Build history of the part. All positions in model axes, mm. Face numbers are marked on the shaded views. A direction names the side the tool comes from. Round coordinates to 2 decimals unless told otherwise and drop trailing zeros. Write each loop counter-clockwise with the first axis right and the second up, starting at its lowest first coordinate (ties: lowest second). Pieces come first, ordered by that corner, then holes. Notation, with made-up numbers: (68, 34) - (108, 34) arc R33 cw to (108, 70) - close; hole circle Ø2 at (14.25, 50.25). An arc over 180 degrees is marked (long way). Answer as a JSON object with one key per item and string values. Group by question number.
Item 1: Probe line 1 (Y direction, x = 9.5, z = 16); line 2 (Z direction, x = 2.25, y = -17.5); line 3 (Z direction, x = 8, y = -4). List the from-to ranges inside material, lowest first. Write a range as from..to.
Item 2: Two-plate mould, pull along Y, no slides. Class the marked faces 3, 4, 5 and 6: +Y half, -Y half, draft (parallel to the pull), parting line (faces both ways), or undercut.
Item 3: Slice it at A-A, the plane z = 16. List the corners of the cut face in (x, y).
Item 4: Which spindle directions (+Z, -Z, +X, -X, +Y, -Y) get a long thin tool onto all of the face, cutting with end or side? Do the marked faces 1 and 2. Say none if no direction does.
Item 5: Flat gauge pins, fed straight in: pin 1 (3.5 mm diameter, centred on x = 7.5, y = -6.5, fed in from +Z); pin 2 (1.5 mm diameter, centred on y = -16, z = -11, fed in from -X). Where does each tip first touch, or does it go through?
Item 6: Slice it at B-B, the plane y = -17. List the corners of the cut face in (x, z).
Item 7: Slice it at D-D, the plane y = 6. List the corners of the cut face in (x, z).
Item 8: Slice it at C-C, the plane x = 6.75. List the corners of the cut face in (y, z).
from build123d import *

# Parameters (mm, degrees)
EXTRUDE_1_DEPTH          = 12.4
CUT_EXTRUDE_1_DEPTH      = 12.1
CUT_EXTRUDE_2_DEPTH      = 21
CUT_EXTRUDE_2_DEPTH_BACK = 16.1
HOLE_WIZARD_M32_D        = 3.4
HOLE_WIZARD_M32_DEPTH    = 15
HOLE_WIZARD_M32_TIP      = 1.021463052
FILLET_2_R               = 1


with BuildPart() as part:
    # Эскиз2 → Бобышка-Вытянуть1 (new body)
    with BuildSketch(Plane(origin=(0, 0, 0), x_dir=(0, 0, -1), z_dir=(1, 0, 0))):
        Polygon((12.1, -8), (12.1, -20), (15.1, -20), (15.1, 10), (-20, 10), (-20, 0), (-3, 0), (-3, -20), (0, -20), (0, -8), align=None)
    extrude(amount=EXTRUDE_1_DEPTH)

    # Эскиз3 → Вырез-Вытянуть1 (cut)
    with BuildSketch(Plane.XY):
        with BuildLine():
            Line((0, 0), (-4.310236897, 0))
            Line((-4.310236897, 0), (-4.310236897, -10.158248203))
            Line((-4.310236897, -10.158248203), (16.784307367, -10.158248203))
            Line((16.784307367, -10.158248203), (16.784307367, 0))
            Line((16.784307367, 0), (12.4, 0))
            ThreePointArc((12.4, 0), (6.2, -6.2), (0, 0))
        make_face()
    extrude(amount=-CUT_EXTRUDE_1_DEPTH, mode=Mode.SUBTRACT)

    # Эскиз4 → Вырез-Вытянуть2 (cut, two sides)
    with BuildSketch(Plane.XY) as cut_extrude_2_sk:
        with BuildLine():
            Line((0, -13.8), (-4.529189241, -13.8))
            Line((-4.529189241, -13.8), (-4.529189241, -23.032738442))
            Line((-4.529189241, -23.032738442), (17.457291493, -23.032738442))
            Line((17.457291493, -23.032738442), (17.457291493, -13.8))
            Line((17.457291493, -13.8), (12.4, -13.8))
            ThreePointArc((12.4, -13.8), (6.2, -20), (0, -13.8))
        make_face()
    extrude(amount=CUT_EXTRUDE_2_DEPTH, mode=Mode.SUBTRACT)
    extrude(cut_extrude_2_sk.sketch, amount=-CUT_EXTRUDE_2_DEPTH_BACK, mode=Mode.SUBTRACT)

    # Отверстие с зазором M32
    with Locations(Plane(origin=(12.4, 0, 0), x_dir=(0, 0, -1), z_dir=(1, 0, 0))):
        with Locations((-6, 5), (-16, 5)):
            Hole(HOLE_WIZARD_M32_D / 2, depth=HOLE_WIZARD_M32_DEPTH)
            with Locations((0, 0, -(HOLE_WIZARD_M32_DEPTH + HOLE_WIZARD_M32_TIP / 2))):  # 118° drill point
                Cone(0, HOLE_WIZARD_M32_D / 2, HOLE_WIZARD_M32_TIP, mode=Mode.SUBTRACT)

    # Эскиз12 → Повернуть1 (revolve)
    with BuildSketch(Plane(origin=(6.2, 0, 0), x_dir=(0, 0, -1), z_dir=(1, 0, 0))):
        with BuildLine():
            Line((12.1, -20), (12.1, -18))
            Line((12.1, -18), (11.3, -18))
            ThreePointArc((11.3, -18), (11.507417596, -19.077032961), (12.1, -20))
        make_face()
    revolve(axis=Axis((6.2, -18, -11.3), (0, 0, -1)))

    # Скругление2
    fillet_2_edges = [part.edges().sort_by_distance(p)[0] for p in [
        (6.2, 10, 20),
    ]]
    fillet(fillet_2_edges, radius=FILLET_2_R)


solid = part.part
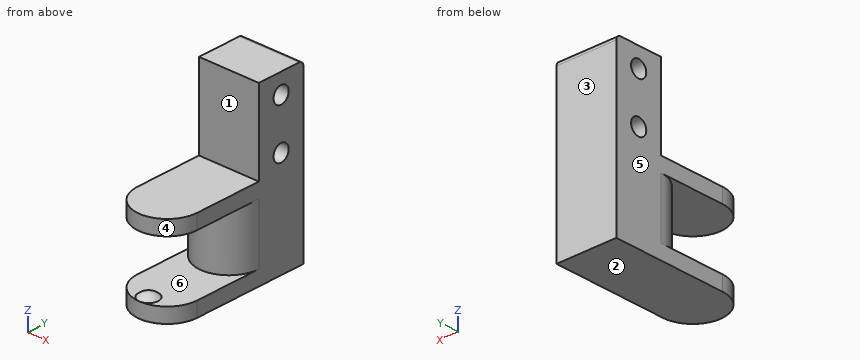
Geometry says:
{
 "1": {"line 1": "y = 0..3.3, 6.7..10", "line 2": "z = -15.1..-12.1, 0..3", "line 3": "z = -15.1..3"},
 "2": {"face 3": "+Y half", "face 4": "-Y half", "face 5": "draft", "face 6": "undercut"},
 "3": {"outline": "(0, 0) - (12.4, 0) - (12.4, 3.3) - (0, 3.3) - close; (0, 6.7) - (12.4, 6.7) - (12.4, 10) - (0, 10) - close"},
 "4": {"face 1": "+Z, +X, -X, -Y", "face 2": "-Z, +X, -X, +Y, -Y"},
 "5": {"pin 1": "stops at z = 3", "pin 2": "passes through"},
 "6": {"outline": "(0.89, -15.1) - (11.51, -15.1) - (11.51, -12.1) - (7.93, -12.1) arc R2.72 ccw to (4.47, -12.1) - (0.89, -12.1) - close; (0.89, 0) - (11.51, 0) - (11.51, 3) - (0.89, 3) - close"},
 "7": {"outline": "(0, -15.1) - (12.4, -15.1) - (12.4, 4.63) - (0, 4.63) - close; (0, 7.37) - (12.4, 7.37) - (12.4, 14.63) - (0, 14.63) - close; (0, 17.37) - (12.4, 17.37) - (12.4, 20) - (0, 20) - close"},
 "8": {"outline": "(-19.98, -15.1) - (10, -15.1) - (10, 19) arc R1 ccw to (9, 20) - (0, 20) - (0, 3) - (-19.98, 3) - (-19.98, 0) - (-6.18, 0) - (-6.18, -12.1) - (-16.08, -12.1) arc R2.85 ccw to (-19.92, -12.1) - (-19.98, -12.1) - close; hole circle Ø3.4 at (5, 6); hole circle Ø3.4 at (5, 16)"}
}
